from build123d import *

# Parameters (mm, degrees)
F2_R      = 1
F3_DEPTH  = 6
F2_R_2    = 1.9
F3_FACE_R = 1
F4_DEPTH  = 2
F5_SIZE   = 0.3
F7_DEPTH  = 1.3


with BuildPart() as f3:
    # F2 (on Top) → F3 (new body)
    with BuildSketch(Plane.XY):
        Circle(F2_R)
    extrude(amount=-F3_DEPTH)

    # F2 (on Top) + F3_face (on face) → F4 (join)
    with BuildSketch(Plane.XY):
        Circle(F2_R_2)
        Circle(F2_R, mode=Mode.SUBTRACT)
    with BuildSketch(Plane.XY):
        Circle(F3_FACE_R)
    extrude(amount=F4_DEPTH)

    # F5
    f5_edges = [f3.edges().sort_by_distance(p)[0] for p in [
        (-1, 0, -6),
        (-1.9, 0, 2),
    ]]
    chamfer(f5_edges, length=F5_SIZE)

    # F6 (on face) → F7 (cut)
    with BuildSketch(Plane.XY.offset(2)):
        Polygon((1, -0.5773502692), (1, 0.5773502692), (0, 1.1547005384), (-1, 0.5773502692), (-1, -0.5773502692), (0, -1.1547005384), align=None)
    extrude(amount=-F7_DEPTH, mode=Mode.SUBTRACT)


solid = f3.part
Verification items for the finished model (mm, model axes). A direction names the side the tool comes from. Round coordinates to 2 decimals unless told otherwise and drop trailing zeros. Loops run counter-clockwise (first coordinate to the right, second up) from the corner with the lowest first, then second, coordinate; pieces in that order, holes last. Notation, with made-up numbers: (77, 57.5) - (86, 57.5) arc R21 cw to (86, 83.5) - close; hole circle Ø8 at (23.5, -5.75). An arc over 180 degrees is marked (long way). Answer in a Markdown table with one row per item. Add a question column.
Q1. Release check for a two-part mould opening along Y. For faces 4 (the face through (-1.9, 0.08, 0.84)), 5 (the face through (0, 0, 0.7)), 6 (the face through (0, 0, -6)) record: pulls with the +Y half, pulls with the -Y half, needs draft (parallel to the pull), parting line crosses it, or undercut.
Q2. Material ranges on line 1 (X direction, y = 0.1, z = 0.75); line 2 (Y direction, x = 0, z = -0.25); line 3 (Z direction, x = -1.2, y = -0.2), recorded low to high.
Q3. Section check A-A on y = 0. Enter the section's corners in (x, z), plus the area to 3 significant figures.
Q4. Section check B-B on z = -3.75. Enter the section's corners in (x, y).
Q5. Gauge pin test, flat ends, axial feed: pin 1 (2 mm diameter, centred on x = -1.5, z = -0.5, fed in from +Y); pin 2 (1.5 mm diameter, centred on x = 1.5, z = 0, fed in from +Y); pin 3 (1.6 mm diameter, centred on x = -0.5, y = 0, fed in from +Z); pin 4 (1.5 mm diameter, centred on y = -1, z = -2.5, fed in from +X). Record the tip position at first contact, or that the pin passes through.
Q6. Tool access check on faces 1 (the face through (-1, 1, 2)), 2 (the face through (1, 0, 1)), 3 (the face through (1, -1, 0)). Record the directions out of +Z, -Z, +X, -X, +Y, -Y that give a thin tool (end or side, any length) a straight path to the whole face; none if there is none.
Found:
| question | item | result |
|---|---|---|
| 1 | face 4 | parting line crosses it |
| 1 | face 5 | undercut |
| 1 | face 6 | needs draft |
| 2 | line 1 | x = -1.9 to -1, 1 to 1.9 |
| 2 | line 2 | y = -1 to 1 |
| 2 | line 3 | z = 0 to 2 |
| 3 | outline | (-1.9, 0) - (-1, 0) - (-1, -5.7) - (-0.7, -6) - (0.7, -6) - (1, -5.7) - (1, 0) - (1.9, 0) - (1.9, 1.7) - (1.6, 2) - (1, 2) - (1, 0.7) - (-1, 0.7) - (-1, 2) - (-1.6, 2) - (-1.9, 1.7) - close |
| 3 | area | 16.8 mm² |
| 4 | outline | circle Ø2 at (0, 0) |
| 5 | pin 1 | stops at y = 1.79 |
| 5 | pin 2 | stops at y = 1.75 |
| 5 | pin 3 | stops at z = 2 |
| 5 | pin 4 | stops at x = 0.97 |
| 6 | face 1 | +Z, +X, -X, +Y, -Y |
| 6 | face 2 | +Z |
| 6 | face 3 | -Z |
